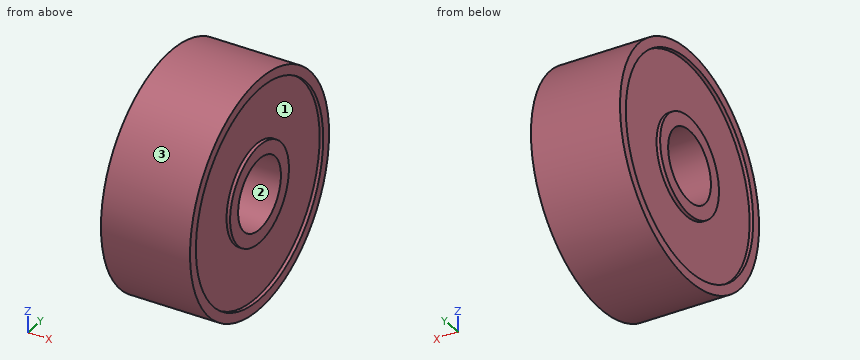
Autodesk Inventor part; units mm, degrees
ref_plane "YZ Plane" through (0, 0, 0) normal (1, 0, 0) x (0, 1, 0)
ref_plane "XZ Plane" through (0, 0, 0) normal (0, 1, 0) x (-1, 0, 0)
ref_plane "XY Plane" through (0, 0, 0) normal (0, 0, 1) x (1, 0, 0)
sketch "Sketch_1" plane through (0, 0, 0) normal (0, 0, 1) x (1, 0, 0)
  line L0 (50, 0) -> (-50, 0)
  line L1 (-2.5, 5.95) -> (-2.3, 5.95)
  line L2 (-2.3, 5.95) -> (-2.3, 2.75)
  line L3 (-2.3, 2.75) -> (-2.5, 2.75)
  line L4 (-2.5, 2.75) -> (-2.5, 2)
  line L5 (-2.5, 2) -> (2.5, 2)
  line L6 (2.5, 2) -> (2.5, 2.75)
  line L7 (2.5, 2.75) -> (2.3, 2.75)
  line L8 (2.3, 2.75) -> (2.3, 5.95)
  line L9 (2.3, 5.95) -> (2.5, 5.95)
  line L10 (2.5, 5.95) -> (2.5, 6.5)
  line L11 (2.5, 6.5) -> (-2.5, 6.5)
  line L12 (-2.5, 6.5) -> (-2.5, 5.95)
revolve "Revolution1" add sketch "Sketch_1" angle 360 about axis through (50, 0, 0) along (1, 0, 0)
properties part number "riku_mae_bis17_624-ZZ-MAE"
Geometry: final body of the model. Coordinates: model frame, mm. Face numbers are marked on the shaded views. Coordinates: 2 decimals unless noted, no trailing zeros. Order: outer loops, then holes, each group sorted by start corner. A loop starts at its lowest first (then second) coordinate and runs counter-clockwise, first axis right, second up. Notation, with made-up numbers: M -14,-23.5 L 45,-23.5 A13 cw 45,-6.5 Z; hole C 56,-38 d10. An arc over 180 degrees is marked long. One line per question, with ' | ' between items. Start each with the question number.
Item 1: Cut plane A-A, the plane y = 0. Return the cut outline in (x, z).
Item 2: Cut plane C-C, the plane x = -2.1. Return the cut outline in (y, z), then the cut area to 3 significant figures.
Item 3: Ray query, probe 1 along Z at (x, y) = (2.45, 0); probe 2 along Z at (x, y) = (0.85, 0); probe 3 along X at (y, z) = (-4.25, -4). Return the intervals inside material, ascending. Write a range as [from, to].
Item 4: Draft query along Y for the marked faces 1, 2 and 3. Return one class per face: released by +Y, released by -Y, zero draft, split by the parting line, or undercut.
Item 5: Pin query (flat end, axial travel): pin 1 Ø1 at (x, z) = (0.5, 2) entering from +Y; pin 2 Ø2 at (x, y) = (1.5, -4.5) entering from +Z; pin 3 Ø1 at (x, y) = (1.5, 2.5) entering from -Z. Return the tip coordinate at first contact, or that it passes through.
Item 6: Cut plane D-D, the plane z = -3.25. Return the cut outline in (x, y), then the cut area to 3 significant figures.
A:
1) outline: M -2.5,-6.5 L 2.5,-6.5 L 2.5,-5.95 L 2.3,-5.95 L 2.3,-2.75 L 2.5,-2.75 L 2.5,-2 L -2.5,-2 L -2.5,-2.75 L -2.3,-2.75 L -2.3,-5.95 L -2.5,-5.95 Z; M -2.5,2 L 2.5,2 L 2.5,2.75 L 2.3,2.75 L 2.3,5.95 L 2.5,5.95 L 2.5,6.5 L -2.5,6.5 L -2.5,5.95 L -2.3,5.95 L -2.3,2.75 L -2.5,2.75 Z
2) outline: C 0,0 d13; hole C 0,0 d4 | area: 120 mm2
3) probe 1: z = [-6.5, -5.95], [-2.75, -2], [2, 2.75], [5.95, 6.5] | probe 2: z = [-6.5, -2], [2, 6.5] | probe 3: x = [-2.3, 2.3]
4) face 1: undercut | face 2: undercut | face 3: split by the parting line
5) pin 1: stops at y = 6.32 | pin 2: stops at z = 5.48 | pin 3: stops at z = -6.18
6) outline: M -2.5,-5.63 L 2.5,-5.63 L 2.5,-4.98 L 2.3,-4.98 L 2.3,4.98 L 2.5,4.98 L 2.5,5.63 L -2.5,5.63 L -2.5,4.98 L -2.3,4.98 L -2.3,-4.98 L -2.5,-4.98 Z | area: 52.3 mm2
